Geometry: final body of the model. Coordinates: model frame, mm. A direction names the side the tool comes from. Give positions to 0.01 mm unless a question says otherwise; leave off trailing zeros. Write each loop counter-clockwise with the first axis right and the second up, starting at its lowest first coordinate (ties: lowest second). Pieces come first, ordered by that corner, then holes. Notation, with made-up numbers: (-37.75, 20.5) - (-27.75, 20.5) arc R33 cw to (-27.75, 58.5) - close; hole circle Ø10 at (75.5, 56.25). An arc over 180 degrees is marked (long way). Return JSON: item names as keys, results as strings.
from build123d import *

# Parameters (mm, degrees)
CROQUIS1_W              = 110
CROQUIS1_H              = 70
SALIENTE_EXTRUIR1_DEPTH = 2
CROQUIS2_W              = 106
CROQUIS2_H              = 66
CROQUIS2_W_2            = 100
CROQUIS2_H_2            = 60
SALIENTE_EXTRUIR2_DEPTH = 10
CROQUIS3_W              = 110
CROQUIS3_H              = 55
CORTAR_EXTRUIR1_DEPTH   = 10
REDONDEO1_START         = -53
REDONDEO1_DEPTH         = 106


with BuildPart() as part:
    # Croquis1 → Saliente-Extruir1 (new body)
    with BuildSketch(Plane(origin=(0, 0, 0), x_dir=(1, 0, 0), z_dir=(0, 1, 0))):
        Rectangle(CROQUIS1_W, CROQUIS1_H)
    extrude(amount=SALIENTE_EXTRUIR1_DEPTH)

    # Croquis2 → Saliente-Extruir2 (add)
    with BuildSketch(Plane(origin=(0, 2, 0), x_dir=(1, 0, 0), z_dir=(0, 1, 0))):
        Rectangle(CROQUIS2_W, CROQUIS2_H)
        Rectangle(CROQUIS2_W_2, CROQUIS2_H_2, mode=Mode.SUBTRACT)
    extrude(amount=SALIENTE_EXTRUIR2_DEPTH)

    # Croquis3 → Cortar-Extruir1 (cut)
    with BuildSketch(Plane(origin=(0, 12, 0), x_dir=(1, 0, 0), z_dir=(0, 1, 0))):
        Rectangle(CROQUIS3_W, CROQUIS3_H)
    extrude(amount=-CORTAR_EXTRUIR1_DEPTH, mode=Mode.SUBTRACT)

    # Redondeo1: read off the stored shape, not the designer's step
    # Redondeo1 outline → Redondeo1 (cut)
    with BuildSketch(Plane.YZ.offset(REDONDEO1_START)):
        with BuildLine():
            Line((4.400657923, -33), (12, -33))
            Line((12, -33), (12, -27.5))
            add(Edge.make_bspline(
                [(12, -27.5), (11.925717186, -27.725800205), (11.717980707, -28.062974077), (11.294012734, -28.57513658), (10.552168001, -29.267993446), (8.343872585, -31.051001592), (6.627785298, -32.237452301), (5.39060754, -32.810235795), (4.741950411, -33), (4.400657923, -33)],
                knots=[0.589454173, 0.589454173, 0.589454173, 0.589454173, 0.589454173, 0.589454173, 1, 1, 1, 1, 1.589454173, 1.589454173, 1.589454173, 1.589454173, 1.589454173, 1.589454173], degree=5, weights=[1, 1, 1.007998589, 1.001618266, 1, 1, 0.973408773, 1.007044093, 1, 1]))
        make_face()
        with BuildLine():
            Line((12, 33), (4.400657923, 33))
            add(Edge.make_bspline(
                [(4.400657923, 33), (4.741950411, 33), (5.39060754, 32.810235795), (6.627785298, 32.237452301), (8.343872585, 31.051001592), (10.552168001, 29.267993446), (11.294012734, 28.57513658), (11.717980707, 28.062974077), (11.925717186, 27.725800205), (12, 27.5)],
                knots=[0, 0, 0, 0, 0, 0, 0.589454173, 0.589454173, 0.589454173, 0.589454173, 1, 1, 1, 1, 1, 1], degree=5, weights=[1, 1, 1.007044093, 0.973408773, 1, 1, 1.001618266, 1.007998589, 1, 1]))
            Line((12, 27.5), (12, 33))
        make_face()
    extrude(amount=REDONDEO1_DEPTH, mode=Mode.SUBTRACT)


solid = part.part
Q1. Section query B-B, the plane z = -16. Return the cut outline in (x, y), plus the area to 3 significant figures.
Answer key:
{"outline": "(-55, 0) - (55, 0) - (55, 2) - (-55, 2) - close", "area": "220 mm^2"}
Q2. Set-up query: faces 1 (the flat face through (53, 6, 30)), 2 (the flat face through (-53, 6, -30)), 3 (the flat face through (-52, 7, -27.5)). Return all of +Z, -Z, +X, -X, +Y, -Y with unobstructed straight access to the full face (end or side cutting, diameter ignored); none if empty.
Answer key:
{"face 1": "+Z, -Z, +X, +Y", "face 2": "+Z, -Z, -X, +Y", "face 3": "+X, -X, +Y"}
Q3. Material intervals for probe 1 along Z at (x, y) = (-38, 4); probe 2 along Y at (x, z) = (8, -27); probe 3 along X at (y, z) = (2.5, -29.5), sorted ascending. Write a range as [from, to].
Answer key:
{"probe 1": "z = [-33, -30], [30, 33]", "probe 2": "y = [0, 2]", "probe 3": "x = [-53, -50], [50, 53]"}
Q4. Pin query (flat end, axial travel): P1, Ø1.3, axis at y = 8, z = -29, coming from the -X side; P2, Ø1, axis at y = 4, z = -10, coming from the +X side; P3, Ø0.9, axis at x = -51, y = 6, coming from the -Z side; P4, Ø3, axis at y = 9, z = 28.5, coming from the +X side. Return the tip coordinate at first contact, or that it passes through.
Answer key:
{"P1": "stops at x = -53", "P2": "passes through", "P3": "stops at z = -32.65", "P4": "stops at x = 53"}
Q5. Mould query, pull axis Z, two halves, no side actions, for faces 4 (the flat face through (-1, 1, -35)), 5 (the flat face through (-50, 7, -29)), 6 (the flat face through (55, 1, 0)). Classes: pulls with the +Z half, pulls with the -Z half, needs draft (parallel to the pull), parting line crosses it, or undercut.
Answer key:
{"face 4": "pulls with the -Z half", "face 5": "undercut", "face 6": "needs draft"}
Q6. Section query A-A, the plane y = 3.25. Return the cut outline in (x, z), plus the area to 3 significant figures.
Answer key:
{"outline": "(-53, -33) - (53, -33) - (53, -27.5) - (50, -27.5) - (50, -30) - (-50, -30) - (-50, -27.5) - (-53, -27.5) - close; (-53, 27.5) - (-50, 27.5) - (-50, 30) - (50, 30) - (50, 27.5) - (53, 27.5) - (53, 33) - (-53, 33) - close", "area": "666 mm^2"}
